```python
from build123d import *

# Parameters (mm, degrees)
SKETCH1_W            = 100
SKETCH1_H            = 65
BOSS_EXTRUDE1_DEPTH  = 1.5
SKETCH2_R            = 3.25
SKETCH2_R_2          = 1.665
BOSS_EXTRUDE2_DEPTH  = 5
SKETCH4_W            = 15
SKETCH4_H            = 10
BOSS_EXTRUDE3_DEPTH  = 1.5
M4_CLEARANCE_HOLE1_D = 4.8
SKETCH8_R            = 3.25
SKETCH8_W            = 55
SKETCH8_H            = 1
SKETCH8_W_2          = 60
BOSS_EXTRUDE4_DEPTH  = 2.5


with BuildPart() as part:
    # Sketch1 → Boss-Extrude1 (new body)
    with BuildSketch(Plane.XY):
        Rectangle(SKETCH1_W, SKETCH1_H)
    extrude(amount=BOSS_EXTRUDE1_DEPTH)

    # Sketch2 → Boss-Extrude2 (add)
    # profile 1 of 4: a face of its own
    with BuildSketch(Plane.XY.offset(1.5)):
        with Locations((-39, 24.5)):
            Circle(SKETCH2_R)
        with Locations((-39, 24.5)):
            Circle(SKETCH2_R_2, mode=Mode.SUBTRACT)
    # profile 2 of 4: a face of its own
    with BuildSketch(Plane.XY.offset(1.5)):
        with Locations((19, 24.5)):
            Circle(SKETCH2_R)
        with Locations((19, 24.5)):
            Circle(SKETCH2_R_2, mode=Mode.SUBTRACT)
    # profile 3 of 4: a face of its own
    with BuildSketch(Plane.XY.offset(1.5)):
        with Locations((19, -24.5)):
            Circle(SKETCH2_R)
        with Locations((19, -24.5)):
            Circle(SKETCH2_R_2, mode=Mode.SUBTRACT)
    # profile 4 of 4: a face of its own
    with BuildSketch(Plane.XY.offset(1.5)):
        with Locations((-39, -24.5)):
            Circle(SKETCH2_R)
        with Locations((-39, -24.5)):
            Circle(SKETCH2_R_2, mode=Mode.SUBTRACT)
    extrude(amount=BOSS_EXTRUDE2_DEPTH)

    # Sketch4 → Boss-Extrude3 (add)
    with BuildSketch(Plane(origin=(0, 0, 0), x_dir=(-1, 0, 0), z_dir=(0, 0, -1))):
        Polygon((-50, -32.5), (-50, -51.5), (-30, -51.5), (-30, -40.5), (30, -40.5), (30, -51.5), (50, -51.5), (50, -32.5), align=None)
        with Locations((-27.5, 37.5)):
            Rectangle(SKETCH4_W, SKETCH4_H)
        with Locations((42.5, 37.5)):
            Rectangle(SKETCH4_W, SKETCH4_H)
    extrude(amount=-BOSS_EXTRUDE3_DEPTH)

    # M4 Clearance Hole1 (through all)
    with Locations(Plane(origin=(0, 0, 0), x_dir=(-1, 0, 0), z_dir=(0, 0, -1))):
        with Locations((-40, -46.5), (40, -46.5), (42.5, 37.5), (-27.5, 37.5)):
            Hole(M4_CLEARANCE_HOLE1_D / 2)

    # Sketch8 → Boss-Extrude4 (add)
    # profile 1 of 3: a face of its own
    with BuildSketch(Plane.XY.offset(1.5)):
        Polygon((-35, 31.5), (-50, 31.5), (-50, -39.5), (-30, -39.5), (30, -39.5), (50, -39.5), (50, 31.5), (35, 31.5), (20, 31.5), align=None)
        with Locations((-39, -24.5)):
            Circle(SKETCH8_R, mode=Mode.SUBTRACT)
        with Locations((19, -24.5)):
            Circle(SKETCH8_R, mode=Mode.SUBTRACT)
        with Locations((-39, 24.5)):
            Circle(SKETCH8_R, mode=Mode.SUBTRACT)
        with Locations((19, 24.5)):
            Circle(SKETCH8_R, mode=Mode.SUBTRACT)
    # profile 2 of 3: a face of its own
    with BuildSketch(Plane.XY.offset(1.5)):
        with Locations((-7.5, 32)):
            Rectangle(SKETCH8_W, SKETCH8_H)
    # profile 3 of 3: a face of its own
    with BuildSketch(Plane.XY.offset(1.5)):
        with Locations((0, -40)):
            Rectangle(SKETCH8_W_2, SKETCH8_H)
    extrude(amount=BOSS_EXTRUDE4_DEPTH)


solid = part.part
```
Source: CAD feature listing. Evaluate the final solid. Frame: model axes, mm. A direction names the side the tool comes from. Round coordinates to 2 decimals unless told otherwise and drop trailing zeros. Write each loop counter-clockwise with the first axis right and the second up, starting at its lowest first coordinate (ties: lowest second). Pieces come first, ordered by that corner, then holes. Notation, with made-up numbers: M 77.25,-10.5 L 96.25,-10.5 A33 cw 96.25,25.5 Z; hole C 69,17 d1. An arc over 180 degrees is marked long. Answer as a JSON object with one key per item and string values. Group by question number.
(1) Reachability of faces 4 (the flat face through (35, 31.5, 3)), 5 (the cylindrical face through (-35.998, -25.745, 5.232)), 6 (the flat face through (42.4, -45.4, 1.5)), 7 (the flat face through (-37.6, 23.1, 6.5)), 8 (the flat face through (-8, 32.5, 2)) from +Z, -Z, +X, -X, +Y, -Y: full face, straight path, thin tool, end or side. Return the list, or none.
(2) Section query A-A on x = 40. Output: boundary loops of the cut face in (y, z), then the cut area to 3 significant figures.
(3) Section query C-C on x = -39. Output: boundary loops of the cut face in (y, z) (3 decimals).
(4) First-contact query: pin 1 (3 mm diameter, centred on x = 27.5, y = 37.5, fed in from -Z); pin 2 (2 mm diameter, centred on x = -11.5, z = 3, fed in from +Y); pin 3 (9.5 mm diameter, centred on x = 38.5, y = -43.5, fed in from +Z); pin 4 (12 mm diameter, centred on x = -43, y = 38, fed in from +Z). Flat tips, straight axial feed; report the tip coordinate or a pass-through.
(5) Section query D-D on x = -26. Output: boundary loops of the cut face in (y, z).
(6) Section query B-B on y = -24.5. Output: boundary loops of the cut face in (x, z) (3 decimals).
(7) Mould query, pull axis Y, two halves, no side actions, for faces 1 (the flat face through (40, -39.5, 3)), 2 (the cylindrical face through (17.679, -25.513, 3.965)), 3 (the flat face through (-42.4, 34.6, 1.5)). Classes: +Y half, -Y half, draft (parallel to the pull), parting line (faces both ways), or undercut.
(8) Ray query, line 1 (Y direction, x = 40, z = 0.9); line 2 (Y direction, x = 27.5, z = 0.35); line 3 (Z direction, x = 39, y = 1). Return the intervals inside material, ascending. Write a range as [from, to].
Computed values:
{
 "1": {"face 4": "+Z, +X, +Y", "face 5": "+Z", "face 6": "+Z, +X, -Y", "face 7": "+Z, +X, -X, +Y, -Y", "face 8": "+Z, -Z, +Y"},
 "2": {"outline": "M -51.5,0 L -48.9,0 L -48.9,1.5 L -51.5,1.5 Z; M -44.1,0 L 32.5,0 L 32.5,1.5 L 31.5,1.5 L 31.5,4 L -39.5,4 L -39.5,1.5 L -44.1,1.5 Z", "area": "296 mm^2"},
 "3": {"outline": "M -51.5,0 L -48.682,0 L -48.682,1.5 L -51.5,1.5 Z; M -44.318,0 L 42.5,0 L 42.5,1.5 L 31.5,1.5 L 31.5,4 L 27.75,4 L 27.75,6.5 L 26.165,6.5 L 26.165,1.5 L 22.835,1.5 L 22.835,6.5 L 21.25,6.5 L 21.25,4 L -21.25,4 L -21.25,6.5 L -22.835,6.5 L -22.835,1.5 L -26.165,1.5 L -26.165,6.5 L -27.75,6.5 L -27.75,4 L -39.5,4 L -39.5,1.5 L -44.318,1.5 Z"},
 "4": {"pin 1": "through", "pin 2": "y = 32.5", "pin 3": "z = 4", "pin 4": "z = 1.5"},
 "5": {"outline": "M -40.5,0 L 32.5,0 L 32.5,4 L -40.5,4 Z"},
 "6": {"outline": "M -50,0 L 50,0 L 50,4 L 22.25,4 L 22.25,6.5 L 20.665,6.5 L 20.665,1.5 L 17.335,1.5 L 17.335,6.5 L 15.75,6.5 L 15.75,4 L -35.75,4 L -35.75,6.5 L -37.335,6.5 L -37.335,1.5 L -40.665,1.5 L -40.665,6.5 L -42.25,6.5 L -42.25,4 L -50,4 Z"},
 "7": {"face 1": "-Y half", "face 2": "undercut", "face 3": "draft"},
 "8": {"line 1": "[-51.5, -48.9], [-44.1, 32.5]", "line 2": "[-40.5, 35.1], [39.9, 42.5]", "line 3": "[0, 4]"}
}
